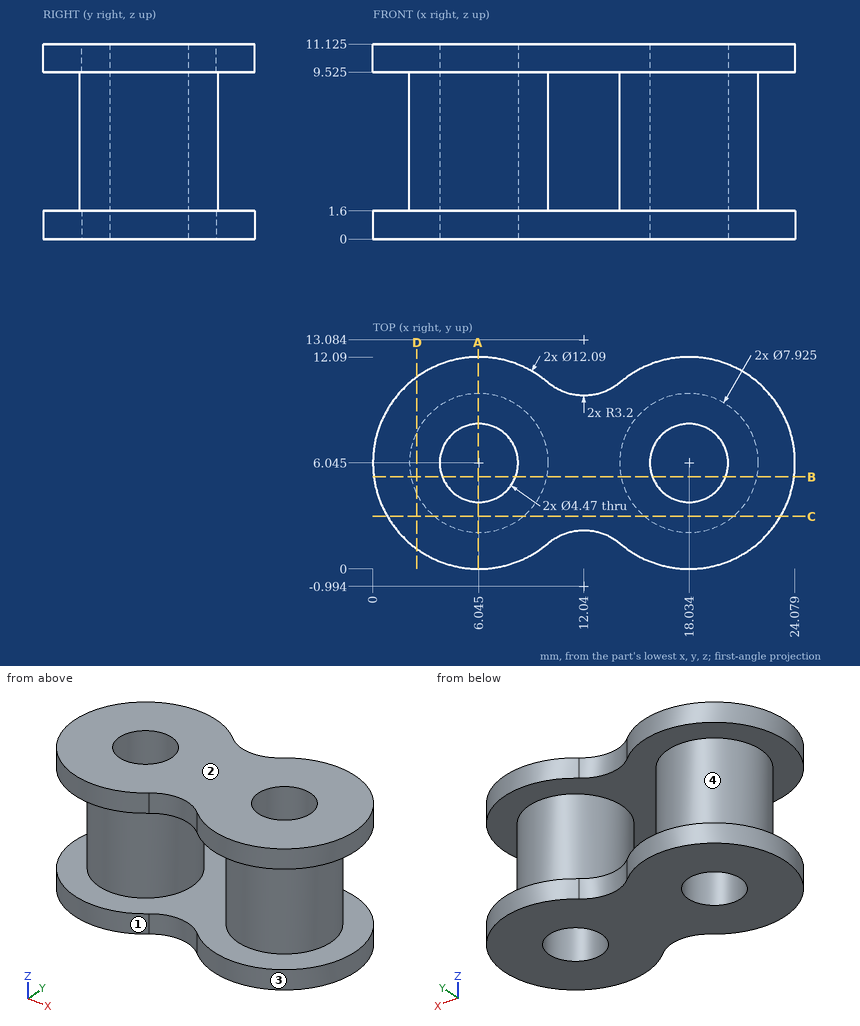
Here's the drawing with two shaded views (mm, measured from the low corner). I have some questions. A direction names the side the tool comes from. Give positions to 0.01 mm unless a question says otherwise; leave off trailing zeros. Write each loop counter-clockwise with the first axis right and the second up, starting at its lowest first coordinate (ties: lowest second). Pieces come first, ordered by that corner, then holes. Notation, with made-up numbers: (78, 83.5) -> (115, 83.5) arc R26 cw to (115, 106.5) -> close; hole circle Ø7 at (-19.5, 88.5). An arc over 180 degrees is marked (long way). Use one line per item in the form item = value. Start each with the question number.
1. Imagine slicing it at D-D on x = 2.5. List the corners of the cut face in (y, z) for me (1 decimal).
2. Will these pins go through, and if not, where does the flat tip stop? pin 1 Ø6 at (x, y) = (9.5, 8) entering from -Z; pin 2 Ø4 at (x, z) = (15, 6.5) entering from -Y; pin 3 Ø2 at (x, z) = (3.5, 7.5) entering from +Y; pin 4 Ø2 at (y, z) = (3.5, 6) entering from -X.
3. On a 3-axis mill with a long thin cutter (end or side, diameter ignored), from which of +Z, -Z, +X, -X, +Y, -Y can I reach the whole of each face in a straight line? I mean the marked faces 3 and 4. Say none if no direction works.
4. Imagine slicing it at B-B on y = 5.25. List the corners of the cut face in (x, z) for me (1 decimal), plus the area to 3 significant figures.
5. Imagine slicing it at C-C on y = 3. List the corners of the cut face in (x, z) for me (1 decimal), plus the area to 3 significant figures.
6. Imagine slicing it at A-A on x = 6. List the corners of the cut face in (y, z) for me (1 decimal).
7. If I drill on L1, parallel to Z at x = 15.5, y = 2 (1 decimal); L2, parallel to X at y = 4.25, z = 8.25 (1 decimal); L3, parallel to X at y = 5.5, z = 1.25 (1 decimal), over which ranges is the centre line in solid material (lowest first)?
8. Thinking about a two-plate mould opening in X: for the marked faces 1 and 2, which applies, +X half, -X half, draft (parallel to the pull), parting line (faces both ways), or undercut?
Entries:
q1.outline = (1.1, 0) -> (10.9, 0) -> (10.9, 1.6) -> (7.8, 1.6) -> (7.8, 9.5) -> (10.9, 9.5) -> (10.9, 11.1) -> (1.1, 11.1) -> (1.1, 9.5) -> (4.3, 9.5) -> (4.3, 1.6) -> (1.1, 1.6) -> close
q2.pin_1 = 0
q2.pin_2 = 2.22
q2.pin_3 = 9.69
q2.pin_4 = 2.4
q3.face_3 = +Z, -Z
q3.face_4 = none
q4.outline = (0.1, 0) -> (4, 0) -> (4, 11.1) -> (0.1, 11.1) -> (0.1, 9.5) -> (2.2, 9.5) -> (2.2, 1.6) -> (0.1, 1.6) -> close; (8.1, 0) -> (15.9, 0) -> (15.9, 11.1) -> (8.1, 11.1) -> close; (20.1, 0) -> (24, 0) -> (24, 1.6) -> (21.9, 1.6) -> (21.9, 9.5) -> (24, 9.5) -> (24, 11.1) -> (20.1, 11.1) -> close; hole (9.9, 1.6) -> (14.2, 1.6) -> (14.2, 9.5) -> (9.9, 9.5) -> close
q4.area = 107 mm²
q5.outline = (0.8, 0) -> (23.3, 0) -> (23.3, 1.6) -> (20.6, 1.6) -> (20.6, 9.5) -> (23.3, 9.5) -> (23.3, 11.1) -> (0.8, 11.1) -> (0.8, 9.5) -> (3.5, 9.5) -> (3.5, 1.6) -> (0.8, 1.6) -> close; hole (8.6, 1.6) -> (15.5, 1.6) -> (15.5, 9.5) -> (8.6, 9.5) -> close
q5.area = 152 mm²
q6.outline = (0, 0) -> (3.8, 0) -> (3.8, 11.1) -> (0, 11.1) -> (0, 9.5) -> (2.1, 9.5) -> (2.1, 1.6) -> (0, 1.6) -> close; (8.3, 0) -> (12.1, 0) -> (12.1, 1.6) -> (10, 1.6) -> (10, 9.5) -> (12.1, 9.5) -> (12.1, 11.1) -> (8.3, 11.1) -> close
q7.L1 = 0 to 1.6, 9.5 to 11.1
q7.L2 = 2.5 to 4.7, 7.4 to 9.6, 14.5 to 16.7, 19.4 to 21.6
q7.L3 = 0 to 3.9, 8.2 to 15.9, 20.2 to 24.1
q8.face_1 = undercut
q8.face_2 = draft
